The model under review builds one solid part; all positions refer to its coordinate system, in mm. Coordinates: 2 decimals unless noted, no trailing zeros. Write each loop counter-clockwise with the first axis right and the second up, starting at its lowest first coordinate (ties: lowest second). Pieces come first, ordered by that corner, then holes.
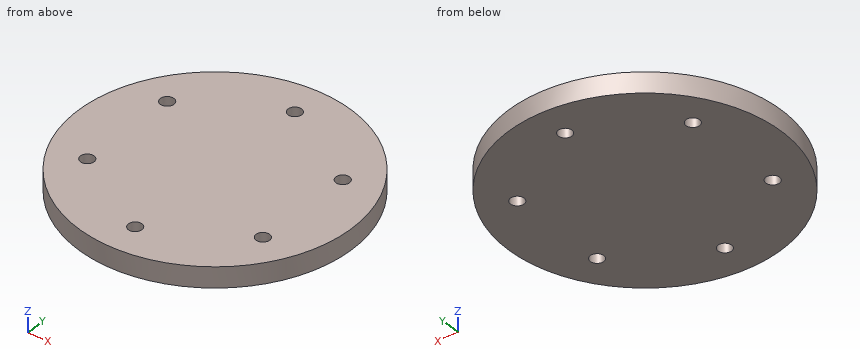
```python
from build123d import *

# Parameters (mm, degrees)
SKETCH1_R           = 40
BOSS_EXTRUDE1_DEPTH = 6
SKETCH2_R           = 2
CUT_EXTRUDE1_DEPTH  = 57.885850613


with BuildPart() as part:
    # Sketch1 → Boss-Extrude1 (new body)
    with BuildSketch(Plane.XY):
        Circle(SKETCH1_R)
    extrude(amount=BOSS_EXTRUDE1_DEPTH)

    # Sketch2 → Cut-Extrude1 (cut, through all)
    with BuildSketch(Plane.XY):
        with Locations((0, 30)):
            Circle(SKETCH2_R)
        with Locations((25.980762114, 15)):
            Circle(SKETCH2_R)
        with Locations((25.980762114, -15)):
            Circle(SKETCH2_R)
        with Locations((0, -30)):
            Circle(SKETCH2_R)
        with Locations((-25.980762114, -15)):
            Circle(SKETCH2_R)
        with Locations((-25.980762114, 15)):
            Circle(SKETCH2_R)
    extrude(amount=CUT_EXTRUDE1_DEPTH, mode=Mode.SUBTRACT)


solid = part.part
```
Item 1: To check wall thickness, follow line 1 along Y through (x, z) = (0, 3.35); line 2 along X through (y, z) = (15, 2.25); line 3 along X through (y, z) = (-31, 2.6). State the ranges of each line that lie inside material, in increasing order.
Solved:
line 1: y = -40 to -32, -28 to 28, 32 to 40
line 2: x = -37.08 to -27.98, -23.98 to 23.98, 27.98 to 37.08
line 3: x = -25.28 to -1.73, 1.73 to 25.28
Item 2: For pin 1 (3 mm diameter, centred on x = 25, z = 3.5, fed in from -Y); pin 2 (2 mm diameter, centred on x = -28.5, z = 5, fed in from -Y); pin 3 (3.5 mm diameter, centred on x = 0, y = 30, fed in from -Z), all flat-tipped, find the tip position at first contact; note any pin that passes through.
Solved:
pin 1: stops at y = -32.37
pin 2: stops at y = -29.05
pin 3: passes through
Item 3: Take a section at A-A, the plane x = 0. Write out the cut boundary in (y, z).
Solved:
outline: (-40, 0) - (-32, 0) - (-32, 6) - (-40, 6) - close; (-28, 0) - (28, 0) - (28, 6) - (-28, 6) - close; (32, 0) - (40, 0) - (40, 6) - (32, 6) - close
Item 4: Take a section at B-B, the plane z = 1. Write out the cut boundary in (x, y).
Solved:
outline: circle Ø80 at (0, 0); hole circle Ø4 at (-25.98, -15); hole circle Ø4 at (-25.98, 15); hole circle Ø4 at (0, -30); hole circle Ø4 at (0, 30); hole circle Ø4 at (25.98, -15); hole circle Ø4 at (25.98, 15)
Item 5: Take a section at D-D, the plane y = -30. Write out the cut boundary in (x, z).
Solved:
outline: (-26.46, 0) - (-2, 0) - (-2, 6) - (-26.46, 6) - close; (2, 0) - (26.46, 0) - (26.46, 6) - (2, 6) - close
Item 6: Take a section at C-C, the plane y = -15. Write out the cut boundary in (x, z).
Solved:
outline: (-37.08, 0) - (-27.98, 0) - (-27.98, 6) - (-37.08, 6) - close; (-23.98, 0) - (23.98, 0) - (23.98, 6) - (-23.98, 6) - close; (27.98, 0) - (37.08, 0) - (37.08, 6) - (27.98, 6) - close
